```python
from build123d import *

# Parameters (mm, degrees)
SKETCH1_R           = 1.5875
SKETCH1_R_2         = 3.175
SKETCH1_R_3         = 1.778
SKETCH1_R_4         = 5.08
BOSS_EXTRUDE1_DEPTH = 6.35


with BuildPart() as part:
    # Sketch1 → Boss-Extrude1 (new body)
    with BuildSketch(Plane.XY):
        Polygon((249.789850187, 155.320558714), (314.789850187, 155.320558714), (314.789850187, -44.679441286), (249.789850187, -44.679441286), (249.789850187, -14.679441286), (179.789850187, -14.679441286), (179.789850187, -44.679441286), (114.789850187, -44.679441286), (114.789850187, 155.320558714), (179.789850187, 155.320558714), (179.789850187, 125.320558714), (249.789850187, 125.320558714), align=None)
        with Locations((140.189850187, -3.099441286)):
            Circle(SKETCH1_R, mode=Mode.SUBTRACT)
        with Locations((122.409850187, 73.100558714)):
            Circle(SKETCH1_R_2, mode=Mode.SUBTRACT)
        with Locations((122.409850187, 37.540558714)):
            Circle(SKETCH1_R_2, mode=Mode.SUBTRACT)
        with Locations((157.969850187, 37.540558714)):
            Circle(SKETCH1_R_2, mode=Mode.SUBTRACT)
        with Locations((140.189850187, 113.740558714)):
            Circle(SKETCH1_R, mode=Mode.SUBTRACT)
        with Locations((157.969850187, 73.100558714)):
            Circle(SKETCH1_R_2, mode=Mode.SUBTRACT)
        with Locations((271.609850187, 73.100558714)):
            Circle(SKETCH1_R_2, mode=Mode.SUBTRACT)
        with Locations((307.169850187, 73.100558714)):
            Circle(SKETCH1_R_2, mode=Mode.SUBTRACT)
        with Locations((271.609850187, 37.540558714)):
            Circle(SKETCH1_R_2, mode=Mode.SUBTRACT)
        with Locations((307.169850187, 37.540558714)):
            Circle(SKETCH1_R_2, mode=Mode.SUBTRACT)
        with Locations((121.139850187, 148.970558714)):
            Circle(SKETCH1_R_2, mode=Mode.SUBTRACT)
        with Locations((140.189850187, 94.677220113)):
            Circle(SKETCH1_R_2, mode=Mode.SUBTRACT)
        with Locations((203.689850187, 94.677220113)):
            Circle(SKETCH1_R_2, mode=Mode.SUBTRACT)
        with Locations((191.294850187, -1.979441286)):
            Circle(SKETCH1_R_3, mode=Mode.SUBTRACT)
        with Locations((197.136850187, -1.979441286)):
            Circle(SKETCH1_R_3, mode=Mode.SUBTRACT)
        with Locations((191.294850187, -8.329441286)):
            Circle(SKETCH1_R_3, mode=Mode.SUBTRACT)
        with Locations((197.136850187, -8.329441286)):
            Circle(SKETCH1_R_3, mode=Mode.SUBTRACT)
        with Locations((191.294850187, 118.970558714)):
            Circle(SKETCH1_R_3, mode=Mode.SUBTRACT)
        with Locations((191.294850187, 112.620558714)):
            Circle(SKETCH1_R_3, mode=Mode.SUBTRACT)
        with Locations((197.136850187, 112.620558714)):
            Circle(SKETCH1_R_3, mode=Mode.SUBTRACT)
        with Locations((197.136850187, 118.970558714)):
            Circle(SKETCH1_R_3, mode=Mode.SUBTRACT)
        with Locations((166.529850187, 79.450558714)):
            Circle(SKETCH1_R_2, mode=Mode.SUBTRACT)
        with Locations((241.459850187, 79.450558714)):
            Circle(SKETCH1_R_2, mode=Mode.SUBTRACT)
        with Locations((166.529850187, 31.190558714)):
            Circle(SKETCH1_R_2, mode=Mode.SUBTRACT)
        with Locations((247.809850187, 31.190558714)):
            Circle(SKETCH1_R_2, mode=Mode.SUBTRACT)
        with Locations((121.139850187, -38.329441286)):
            Circle(SKETCH1_R_2, mode=Mode.SUBTRACT)
        with Locations((308.439850187, -38.329441286)):
            Circle(SKETCH1_R_2, mode=Mode.SUBTRACT)
        with Locations((308.439850187, 148.970558714)):
            Circle(SKETCH1_R_2, mode=Mode.SUBTRACT)
        with Locations((165.076665974, 118.820558714)):
            Circle(SKETCH1_R_4, mode=Mode.SUBTRACT)
        with Locations((165.076665974, -8.179441286)):
            Circle(SKETCH1_R_4, mode=Mode.SUBTRACT)
        with BuildLine():
            Line((135.109850187, 24.840558714), (294.469850187, 24.840558714))
            ThreePointArc((294.469850187, 24.840558714), (303.359850187, 15.950558714), (294.469850187, 7.060558714))
            Line((294.469850187, 7.060558714), (135.109850187, 7.060558714))
            ThreePointArc((135.109850187, 7.060558714), (126.219850187, 15.950558714), (135.109850187, 24.840558714))
        make_face(mode=Mode.SUBTRACT)
        with BuildLine():
            Line((218.269850187, 103.580558714), (294.469850187, 103.580558714))
            ThreePointArc((294.469850187, 103.580558714), (303.359850187, 94.690558714), (294.469850187, 85.800558714))
            Line((294.469850187, 85.800558714), (218.269850187, 85.800558714))
            ThreePointArc((218.269850187, 85.800558714), (209.379850187, 94.690558714), (218.269850187, 103.580558714))
        make_face(mode=Mode.SUBTRACT)
    extrude(amount=BOSS_EXTRUDE1_DEPTH)


solid = part.part
```
Could you check a few things on this model? Use its own coordinates, in mm. A direction names the side the tool comes from. Give positions to 0.01 mm unless a question says otherwise; leave off trailing zeros. Order: outer loops, then holes, each group sorted by start corner. A loop starts at its lowest first (then second) coordinate and runs counter-clockwise, first axis right, second up.
Q1. Suppose I cut it at C-C, the plane x = 221. Write out the boundary of the cut face in (y, z).
Q2. For faces 1 (the flat face through (283, -44.679, 3)), 2 (the cylindrical face through (209.38, 94.5, 3.13)), which set-ups out of +Z, -Z, +X, -X, +Y, -Y let a thin tool reach every point of the face, with its end or its side?
Q3. Suppose I cut it at A-A, the plane y = -17.5. Write out the boundary of the cut face in (x, z).
Q4. Suppose I cut it at B-B, the plane x = 174. Write out the boundary of the cut face in (y, z), and give its area (3 significant figures).
Q5. Suppose I cut it at D-D, the plane x = 272.5. Write out the boundary of the cut face in (y, z).
Q6. We'd pull the mould along Y, two halves only. Please class faces 3 (the flat face through (215, -14.679, 3)), 4 (the flat face through (282, 155.321, 3)), 5 (the cylindrical face through (238.94, 77.52, 3.13)): +Y half, -Y half, draft (parallel to the pull), parting line (faces both ways), or undercut.
Q7. I'm going to push a flat-ended pin straight in: P1, Ø2, axis at x = 225, z = 2, coming from the +Y side. Where does the tip first touch, or does it pass through?
Q8. If I drill on line 1 along Y through (x, z) = (271.5, 6); line 2 along Y through (x, z) = (262, 2.5); line 3 along Y through (x, z) = (140, 1), over which ranges is the centre line in solid material (lowest first)?
Solution:
1. outline: (-14.68, 0) - (7.06, 0) - (7.06, 6.35) - (-14.68, 6.35) - close; (24.84, 0) - (85.8, 0) - (85.8, 6.35) - (24.84, 6.35) - close; (103.58, 0) - (125.32, 0) - (125.32, 6.35) - (103.58, 6.35) - close
2. face 1: +Z, -Z, +X, -X, -Y
2. face 2: +Z, -Z
3. outline: (114.79, 0) - (179.79, 0) - (179.79, 6.35) - (114.79, 6.35) - close; (249.79, 0) - (314.79, 0) - (314.79, 6.35) - (249.79, 6.35) - close
4. outline: (-44.68, 0) - (7.06, 0) - (7.06, 6.35) - (-44.68, 6.35) - close; (24.84, 0) - (155.32, 0) - (155.32, 6.35) - (24.84, 6.35) - close
4. area: 1,160 mm2
5. outline: (-44.68, 0) - (7.06, 0) - (7.06, 6.35) - (-44.68, 6.35) - close; (24.84, 0) - (34.49, 0) - (34.49, 6.35) - (24.84, 6.35) - close; (40.59, 0) - (70.05, 0) - (70.05, 6.35) - (40.59, 6.35) - close; (76.15, 0) - (85.8, 0) - (85.8, 6.35) - (76.15, 6.35) - close; (103.58, 0) - (155.32, 0) - (155.32, 6.35) - (103.58, 6.35) - close
6. face 3: -Y half
6. face 4: +Y half
6. face 5: undercut
7. P1: stops at y = 125.32
8. line 1: y = -44.68 to 7.06, 24.84 to 34.37, 40.71 to 69.93, 76.27 to 85.8, 103.58 to 155.32
8. line 2: y = -44.68 to 7.06, 24.84 to 85.8, 103.58 to 155.32
8. line 3: y = -44.68 to -4.68, -1.52 to 7.06, 24.84 to 91.51, 97.85 to 112.16, 115.32 to 155.32
